```python
from build123d import *

# Parameters (mm, degrees)
SKETCH1_W           = 85.5
SKETCH1_H           = 41
BOSS_EXTRUDE1_DEPTH = 40
SKETCH2_W           = 4.5
SKETCH2_H           = 41
BOSS_EXTRUDE2_DEPTH = 4.8
SKETCH5_W           = 81.5
SKETCH5_H           = 37.5
CUT_EXTRUDE1_DEPTH  = 10
SKETCH6_W           = 45
SKETCH6_H           = 5
CUT_EXTRUDE2_DEPTH  = 25
SKETCH7_W           = 71.5
SKETCH7_H           = 27.5
CUT_EXTRUDE3_DEPTH  = 25
CUT_EXTRUDE4_REACH  = 60.931
SKETCH10_W          = 22
SKETCH10_H          = 28


with BuildPart() as part:
    # Sketch1 → Boss-Extrude1 (new body)
    with BuildSketch(Plane(origin=(0, 0, 0), x_dir=(1, 0, 0), z_dir=(0, 1, 0))):
        Rectangle(SKETCH1_W, SKETCH1_H)
    extrude(amount=BOSS_EXTRUDE1_DEPTH)

    # Sketch2 → Boss-Extrude2 (add)
    with BuildSketch(Plane.XZ):
        with Locations((-6.65, 0)):
            Rectangle(SKETCH2_W, SKETCH2_H)
        with Locations((6.65, 0)):
            Rectangle(SKETCH2_W, SKETCH2_H)
    extrude(amount=BOSS_EXTRUDE2_DEPTH)

    # Sketch5 → Cut-Extrude1 (cut)
    with BuildSketch(Plane(origin=(0, 40, 0), x_dir=(1, 0, 0), z_dir=(0, 1, 0))):
        Rectangle(SKETCH5_W, SKETCH5_H)
    extrude(amount=-CUT_EXTRUDE1_DEPTH, mode=Mode.SUBTRACT)

    # Sketch6 → Cut-Extrude2 (cut)
    with BuildSketch(Plane(origin=(0, 30, 0), x_dir=(1, 0, 0), z_dir=(0, 1, 0))):
        with Locations((-13.25, 16.25)):
            Rectangle(SKETCH6_W, SKETCH6_H)
        with Locations((13.25, -16.25)):
            Rectangle(SKETCH6_W, SKETCH6_H)
    extrude(amount=-CUT_EXTRUDE2_DEPTH, mode=Mode.SUBTRACT)

    # Sketch7 → Cut-Extrude3 (cut)
    with BuildSketch(Plane(origin=(0, 30, 0), x_dir=(1, 0, 0), z_dir=(0, 1, 0))):
        Rectangle(SKETCH7_W, SKETCH7_H)
    extrude(amount=-CUT_EXTRUDE3_DEPTH, mode=Mode.SUBTRACT)

    # Sketch10 → Cut-Extrude4 (cut, up to next)
    with BuildSketch(Plane(origin=(0, 5, 0), x_dir=(1, 0, 0), z_dir=(0, 1, 0)), mode=Mode.PRIVATE) as cut_extrude4_sk1:
        with Locations((-22.406521178, 2.5)):
            Rectangle(SKETCH10_W, SKETCH10_H)
    cut_extrude4_tool1 = extrude(cut_extrude4_sk1.sketch, amount=-CUT_EXTRUDE4_REACH, mode=Mode.PRIVATE) & part.part
    # Sketch10 → Cut-Extrude4 (cut, up to next)
    with BuildSketch(Plane(origin=(0, 5, 0), x_dir=(1, 0, 0), z_dir=(0, 1, 0)), mode=Mode.PRIVATE) as cut_extrude4_sk2:
        with Locations((22.4125, -2.5)):
            Rectangle(SKETCH10_W, SKETCH10_H)
    cut_extrude4_tool2 = extrude(cut_extrude4_sk2.sketch, amount=-CUT_EXTRUDE4_REACH, mode=Mode.PRIVATE) & part.part
    add(cut_extrude4_tool1.solids().sort_by_distance((-22.406521, 5, -2.5))[0], mode=Mode.SUBTRACT)
    add(cut_extrude4_tool2.solids().sort_by_distance((22.4125, 5, 2.5))[0], mode=Mode.SUBTRACT)


solid = part.part
```
Source: CAD feature listing. Evaluate the final solid. Frame: model axes, mm. A direction names the side the tool comes from. Round coordinates to 2 decimals unless told otherwise and drop trailing zeros. Order: outer loops, then holes, each group sorted by start corner. A loop starts at its lowest first (then second) coordinate and runs counter-clockwise, first axis right, second up. Notation, with made-up numbers: (9, -18) -> (21, -18) arc R35 cw to (21, 16) -> close; hole circle Ø7 at (4.5, 42.25). An arc over 180 degrees is marked (long way). One line per item, written item: value. Start each with the question number.
Q1. Section query C-C (y = 7). Return the cut outline in (x, z), plus the area to 3 significant figures.
Q2. Draft query along Z for faces 4 (the flat face through (8.9, -2, 0)), 5 (the flat face through (33.412, 3, 3)). Return one class per face: pulls with the +Z half, pulls with the -Z half, needs draft (parallel to the pull), parting line crosses it, or undercut.
Q3. Material intervals for probe 1 along X at (y, z) = (0.5, -9); probe 2 along X at (y, z) = (18, 18); probe 3 along Z at (x, y) = (-7.5, 14.5), sorted ascending.
Q4. Pin query (flat end, axial travel): pin 1 (11 mm diameter, centred on x = 12, z = -6, fed in from +Y); pin 2 (5.5 mm diameter, centred on y = -3, z = 1, fed in from +X). Return the tip coordinate at first contact, or that it passes through.
Q5. Section query A-A (z = -15). Return the cut outline in (x, y), plus the area to 3 significant figures.
Q6. Section query B-B (x = -24). Return the cut outline in (y, z).
Q7. Section query D-D (z = -4.5). Return the cut outline in (x, y), plus the area to 3 significant figures.
Q8. Access query for faces 1 (the flat face through (-23, 18, 13.75)), 2 (the flat face through (-8.9, -2, 0)), 3 (the flat face through (-4.4, -2, 0)). Directions: +Z, -Z, +X, -X, +Y, -Y. A direction counts if a zero-diameter tool reaches every point of the face in a straight line with its end or side. Return the directions, or none.
Findings below:
1. outline: (-42.75, -20.5) -> (42.75, -20.5) -> (42.75, 20.5) -> (-42.75, 20.5) -> close; hole (-35.75, -18.75) -> (9.25, -18.75) -> (9.25, -13.75) -> (35.75, -13.75) -> (35.75, 18.75) -> (-9.25, 18.75) -> (-9.25, 13.75) -> (-35.75, 13.75) -> close
1. area: 1,090 mm²
2. face 4: needs draft
2. face 5: undercut
3. probe 1: -42.75 to -33.41, -11.41 to 11.41, 33.41 to 42.75
3. probe 2: -42.75 to -9.25, 35.75 to 42.75
3. probe 3: -20.5 to -18.75, 18.75 to 20.5
4. pin 1: y = 5
4. pin 2: x = 8.9
5. outline: (-42.75, 0) -> (-33.41, 0) -> (-33.41, 5) -> (-35.75, 5) -> (-35.75, 30) -> (-40.75, 30) -> (-40.75, 40) -> (-42.75, 40) -> close; (-11.41, 0) -> (-8.9, 0) -> (-8.9, -4.8) -> (-4.4, -4.8) -> (-4.4, 0) -> (4.4, 0) -> (4.4, -4.8) -> (8.9, -4.8) -> (8.9, 0) -> (42.75, 0) -> (42.75, 40) -> (40.75, 40) -> (40.75, 30) -> (9.25, 30) -> (9.25, 5) -> (-11.41, 5) -> close
5. area: 1,410 mm²
6. outline: (0, -20.5) -> (40, -20.5) -> (40, -18.75) -> (5, -18.75) -> (5, -16.5) -> (0, -16.5) -> close; (0, 11.5) -> (5, 11.5) -> (5, 13.75) -> (30, 13.75) -> (30, 18.75) -> (40, 18.75) -> (40, 20.5) -> (0, 20.5) -> close
7. outline: (-42.75, 0) -> (-33.41, 0) -> (-33.41, 5) -> (-35.75, 5) -> (-35.75, 30) -> (-40.75, 30) -> (-40.75, 40) -> (-42.75, 40) -> close; (-11.41, 0) -> (-8.9, 0) -> (-8.9, -4.8) -> (-4.4, -4.8) -> (-4.4, 0) -> (4.4, 0) -> (4.4, -4.8) -> (8.9, -4.8) -> (8.9, 0) -> (11.41, 0) -> (11.41, 5) -> (-11.41, 5) -> close; (33.41, 0) -> (42.75, 0) -> (42.75, 40) -> (40.75, 40) -> (40.75, 30) -> (35.75, 30) -> (35.75, 5) -> (33.41, 5) -> close
7. area: 641 mm²
8. face 1: +Y
8. face 2: +Z, -Z, -X, -Y
8. face 3: +Z, -Z, -Y
